```python
from build123d import *

# Parameters (mm, degrees)
BOSS_EXTRUDE1_DEPTH = 304.8
SKETCH2_R           = 6.35
CUT_EXTRUDE1_DEPTH  = 599.68125614


with BuildPart() as part:
    # Sketch1 → Boss-Extrude1 (new body)
    with BuildSketch(Plane(origin=(0, 0, 0), x_dir=(1, 0, 0), z_dir=(0, 1, 0))):
        Polygon((3.175, 2.097530582), (595.50625614, 2.097530582), (595.50625614, -53.975), (598.68125614, -53.975), (598.68125614, 0), (598.68125614, 5.272530582), (0, 5.272530582), (0, 0), (0, -53.975), (3.175, -53.975), align=None)
    extrude(amount=BOSS_EXTRUDE1_DEPTH)

    # Sketch2 → Cut-Extrude1 (cut, through all)
    with BuildSketch(Plane.ZY):
        with Locations((24.351234709, 152.4)):
            Circle(SKETCH2_R)
    extrude(amount=-CUT_EXTRUDE1_DEPTH, mode=Mode.SUBTRACT)


solid = part.part
```
Build history of the part. All positions in model axes, mm. A direction names the side the tool comes from. Round coordinates to 2 decimals unless told otherwise and drop trailing zeros. Write each loop counter-clockwise with the first axis right and the second up, starting at its lowest first coordinate (ties: lowest second). Pieces come first, ordered by that corner, then holes.
1) Pin check, flat tips, straight feed: pin 1 (16.5 mm diameter, centred on y = 152.4, z = 24.35, fed in from +X); pin 2 (10 mm diameter, centred on y = 152.4, z = 24.35, fed in from -X). Stop position of each tip, or through.
2) 3-axis set-ups, long thin cutter, end or side, ignore diameter. For faces 1 (the flat face through (3.175, 150, 33)), 2 (the flat face through (298, 304.8, -4)): which of +Z, -Z, +X, -X, +Y, -Y reach the whole face in a straight line?
3) Mould opens along Y. For faces 3 (the flat face through (298, 0, -4)), 4 (the cylindrical face through (1.565, 158.696, 23.525)), 5 (the flat face through (595.506, 150, 32)) say: +Y half, -Y half, draft (parallel to the pull), parting line (faces both ways), or undercut.
4) Band-saw the part on B-B, the plane y = 152.4. List the corners of the cut face in (x, z) (3 decimals).
5) Band-saw the part on C-C, the plane x = 244. List the corners of the cut face in (y, z).
6) Band-saw the part on D-D, the plane y = 280. List the corners of the cut face in (x, z) (3 decimals), and give its area (3 significant figures).
7) Band-saw the part on A-A, the plane z = 43.5. List the corners of the cut face in (x, y) (3 decimals).
8) Drill centre lines: probe 1 along Z at (x, y) = (596, 152) (3 decimals); probe 2 along X at (y, z) = (121, 19) (3 decimals); probe 3 along Z at (x, y) = (44.5, 174). Where is each one in solid material? Low to high.
Ans:
1. pin 1: stops at x = 598.68
1. pin 2: passes through
2. face 1: +Z, +Y, -Y
2. face 2: +Z, -Z, +X, -X, +Y
3. face 3: -Y half
3. face 4: undercut
3. face 5: draft
4. outline: (0, -5.273) - (598.681, -5.273) - (598.681, 18.001) - (595.506, 18.001) - (595.506, -2.098) - (3.175, -2.098) - (3.175, 18.001) - (0, 18.001) - close; (0, 30.701) - (3.175, 30.701) - (3.175, 53.975) - (0, 53.975) - close; (595.506, 30.701) - (598.681, 30.701) - (598.681, 53.975) - (595.506, 53.975) - close
5. outline: (0, -5.27) - (304.8, -5.27) - (304.8, -2.1) - (0, -2.1) - close
6. outline: (0, -5.273) - (598.681, -5.273) - (598.681, 53.975) - (595.506, 53.975) - (595.506, -2.098) - (3.175, -2.098) - (3.175, 53.975) - (0, 53.975) - close
6. area: 2,260 mm2
7. outline: (0, 0) - (3.175, 0) - (3.175, 304.8) - (0, 304.8) - close; (595.506, 0) - (598.681, 0) - (598.681, 304.8) - (595.506, 304.8) - close
8. probe 1: z = -5.273 to 18.014, 30.689 to 53.975
8. probe 2: x = 0 to 3.175, 595.506 to 598.681
8. probe 3: z = -5.27 to -2.1
